Here's how the part is built. I have some questions about the finished solid (model axes, mm). A direction names the side the tool comes from. Give positions to 0.01 mm unless a question says otherwise; leave off trailing zeros. Loops run counter-clockwise (first coordinate to the right, second up) from the corner with the lowest first, then second, coordinate; pieces in that order, holes last. Notation, with made-up numbers: (-36, 61) - (-18, 61) arc R23 cw to (-18, 82) - close; hole circle Ø8 at (9, 32). An arc over 180 degrees is marked (long way). Return JSON: item names as keys, results as strings. Group by question number.
(1) On a 3-axis mill with a long thin cutter (end or side, diameter ignored), from which of +Z, -Z, +X, -X, +Y, -Y can I reach the whole of each face in a straight line? I mean faces 5 (the flat face through (-68, 2.736, 9)), 6 (the flat face through (-75, 20, -5.5)), 7 (the flat face through (-70, 21, 15)), 8 (the flat face through (-70, 14.113, 23)), 9 (the flat face through (-72, 15, 18)). Say none if no direction works.
(2) If we section it at C-C (x = -83): Please give me the cut outline in (y, z).
(3) If we section it at A-A (z = 22): Please give me the cut outline in (x, y), then the cut area to 3 significant figures.
(4) If we section it at B-B (z = 16): Please give me the cut outline in (x, y), then the cut area to 3 significant figures.
(5) If we mould it in two halves opening along X, with no side actions, what happens to faces 1 (the flat face through (-65, 20, -5.5)), 2 (the flat face through (-72.3, 12.5, -1.5)), 3 (the flat face through (-73.543, 18, 23)), 4 (the cylindrical face through (-70.06, 12.62, 25.28))? For each: released by +X, released by -X, zero draft, split by the parting line, or undercut.
(6) I need wall thicknesses on probe 1 along Z at (x, y) = (-58.5, 15); probe 2 along Z at (x, y) = (-70.5, 17); probe 3 along X at (y, z) = (16, 22.5). Which ranges of each line are inside material? Lowest first, please. Write a range as [from, to].
(7) For P1, Ø6, axis at y = 15.5, z = -1.5, coming from the +X side; P2, Ø2, axis at x = -67, y = 18.5, coming from the -Z side; P3, Ø1.8, axis at y = 4.5, z = 7, coming from the +X side, each with a flat end and sliding along its axis, tell me the tip position at first contact or that it passes through.
(8) If we section it at D-D (x = -65): State how many separate pieces and enclosed holes the cut face has, then the cut area to 3 significant figures.
```python
from build123d import *

# Parameters (mm, degrees)
SALIENTE_EXTRUIR1_DEPTH = 18
SALIENTE_EXTRUIR2_START = 1.5
CROQUIS2_R              = 2.7
SALIENTE_EXTRUIR2_DEPTH = 1.5
SALIENTE_EXTRUIR3_DEPTH = 1.5
CROQUIS6_W              = 5.4
CROQUIS6_H              = 1.803822617
SALIENTE_EXTRUIR7_DEPTH = 10
CROQUIS10_W             = 5.4
CROQUIS10_H             = 10
CORTAR_EXTRUIR3_DEPTH   = 10
CROQUIS12_W             = 50.345864286
CROQUIS12_H             = 43.398115734
CORTAR_EXTRUIR4_DEPTH   = 30
CROQUIS14_W             = 2
CROQUIS14_H             = 3
CORTAR_EXTRUIR5_DEPTH   = 30
CORTAR_EXTRUIR7_START   = -7.4
CROQUIS16_W             = 3
CROQUIS16_H             = 7.002646448
CROQUIS16_H_2           = 3.270183245
CORTAR_EXTRUIR7_DEPTH   = 7.4
CROQUIS17_W             = 3.7
CROQUIS17_H             = 3
REVOLUCI_N2_ANGLE       = 180
CROQUIS19_W             = 0.5
CROQUIS19_H             = 9
REVOLUCI_N3_ANGLE       = 180


with BuildPart() as part:
    # Croquis1 → Saliente-Extruir1 (new body)
    with BuildSketch(Plane.XY):
        with BuildLine():
            Line((-53.667784589, 33.4650382), (-54.417784589, 34.764076306))
            Line((-54.417784589, 34.764076306), (-59.613937012, 31.764076306))
            ThreePointArc((-59.613937012, 31.764076306), (-73.945502317, 40.827707086), (-87.584573208, 30.752047693))
            Line((-87.584573208, 30.752047693), (-88.334573208, 29.453009587))
            Line((-88.334573208, 29.453009587), (-83.138420786, 26.453009587))
            ThreePointArc((-83.138420786, 26.453009587), (-83.82197264, 9.509694567), (-68.276660199, 2.735742387))
            Line((-68.276660199, 2.735742387), (-66.776660199, 2.735742387))
            Line((-66.776660199, 2.735742387), (-66.776660199, 8.735742387))
            ThreePointArc((-66.776660199, 8.735742387), (-51.761543041, 16.615426627), (-53.667784589, 33.4650382))
        make_face()
        with BuildLine():
            Line((-54.507549641, 31.745180452), (-55.016343575, 32.626437397))
            Line((-55.016343575, 32.626437397), (-60.212495998, 29.626437397))
            ThreePointArc((-60.212495998, 29.626437397), (-72.508207296, 39.071771198), (-85.675250182, 30.884718699))
            Line((-85.675250182, 30.884718699), (-86.184044116, 30.003461754))
            Line((-86.184044116, 30.003461754), (-80.987891693, 27.003461754))
            ThreePointArc((-80.987891693, 27.003461754), (-83.019935064, 11.632396511), (-69.346218174, 4.322929129))
            Line((-69.346218174, 4.322929129), (-68.328630306, 4.322929129))
            Line((-68.328630306, 4.322929129), (-68.328630306, 10.322929129))
            ThreePointArc((-68.328630306, 10.322929129), (-54.000875637, 16.248660571), (-54.507549641, 31.745180452))
        make_face(mode=Mode.SUBTRACT)
    extrude(amount=SALIENTE_EXTRUIR1_DEPTH)

    # Croquis2 → Saliente-Extruir2 (add)
    with BuildSketch(Plane(origin=(0, 0, 0), x_dir=(-1, 0, 0), z_dir=(0, 0, -1)).offset(SALIENTE_EXTRUIR2_START)):
        with BuildLine():
            Line((87.584573208, 30.752047693), (88.334573208, 29.453009587))
            Line((88.334573208, 29.453009587), (83.138420786, 26.453009587))
            ThreePointArc((83.138420786, 26.453009587), (83.82197264, 9.509694567), (68.276660199, 2.735742387))
            Line((68.276660199, 2.735742387), (66.776660199, 2.735742387))
            Line((66.776660199, 2.735742387), (66.776660199, 8.735742387))
            ThreePointArc((66.776660199, 8.735742387), (51.761543041, 16.615426627), (53.667784589, 33.4650382))
            Line((53.667784589, 33.4650382), (54.417784589, 34.764076306))
            Line((54.417784589, 34.764076306), (59.613937012, 31.764076306))
            ThreePointArc((59.613937012, 31.764076306), (73.945502317, 40.827707086), (87.584573208, 30.752047693))
        make_face()
        with Locations((69.843005999, 22.317609427)):
            Circle(CROQUIS2_R, mode=Mode.SUBTRACT)
    extrude(amount=-SALIENTE_EXTRUIR2_DEPTH)

    # Croquis3 → Saliente-Extruir3 (add)
    with BuildSketch(Plane.XY.offset(18)):
        with BuildLine():
            Line((-66.776660199, 8.735742387), (-66.776660199, 2.735742387))
            Line((-66.776660199, 2.735742387), (-68.276660199, 2.735742387))
            ThreePointArc((-68.276660199, 2.735742387), (-83.82197264, 9.509694567), (-83.138420786, 26.453009587))
            Line((-83.138420786, 26.453009587), (-88.334573208, 29.453009587))
            Line((-88.334573208, 29.453009587), (-87.584573208, 30.752047693))
            ThreePointArc((-87.584573208, 30.752047693), (-73.945502317, 40.827707086), (-59.613937012, 31.764076306))
            Line((-59.613937012, 31.764076306), (-54.417784589, 34.764076306))
            Line((-54.417784589, 34.764076306), (-53.667784589, 33.4650382))
            ThreePointArc((-53.667784589, 33.4650382), (-51.761543041, 16.615426627), (-66.776660199, 8.735742387))
        make_face()
    extrude(amount=SALIENTE_EXTRUIR3_DEPTH)

    # Croquis6 → Saliente-Extruir7 (add)
    with BuildSketch(Plane(origin=(0, 0, -1.5), x_dir=(-1, 0, 0), z_dir=(0, 0, -1))):
        with Locations((69.843005999, 21.415698119)):
            Rectangle(CROQUIS6_W, CROQUIS6_H)
    extrude(amount=SALIENTE_EXTRUIR7_DEPTH)

    # Croquis10 → Cortar-Extruir3 (cut)
    with BuildSketch(Plane(origin=(0, 22.317609427, 0), x_dir=(1, 0, 0), z_dir=(0, 1, 0))):
        with Locations((-69.843005999, 6.5)):
            Rectangle(CROQUIS10_W, CROQUIS10_H)
    extrude(amount=-CORTAR_EXTRUIR3_DEPTH, mode=Mode.SUBTRACT)

    # Croquis11 → Revolución1 (revolve)
    with BuildSketch(Plane(origin=(0, 22.317609427, 0), x_dir=(1, 0, 0), z_dir=(0, 1, 0)), mode=Mode.PRIVATE) as revoluci_n1_sk:
        Polygon((-72.543005999, 1.5), (-79.543005999, 1.5), (-72.543005999, 11.5), align=None)
        Polygon((-71.193005999, -19.5), (-69.843005999, -19.5), (-69.843005999, -26.5), (-71.193005999, -26.5), (-79.543005999, -26.5), (-79.543005999, -19.5), align=None)
    revolve(revoluci_n1_sk.sketch.rotate(Axis((-69.843005999, 22.317609427, 19.5), (0, 0, 1)), 180), axis=Axis((-69.843005999, 22.317609427, 19.5), (0, 0, 1)))

    # Croquis12 → Cortar-Extruir4 (cut)
    with BuildSketch(Plane(origin=(0, 22.317609427, 0), x_dir=(1, 0, 0), z_dir=(0, 1, 0))):
        with Locations((-66.462924906, -7.850212976)):
            Rectangle(CROQUIS12_W, CROQUIS12_H)
    extrude(amount=CORTAR_EXTRUIR4_DEPTH, mode=Mode.SUBTRACT)

    # Croquis14 → Cortar-Extruir5 (cut)
    with BuildSketch(Plane(origin=(0, 22.317609427, 0), x_dir=(-1, 0, 0), z_dir=(0, 1, 0))):
        with Locations((65.143005999, -4)):
            Rectangle(CROQUIS14_W, CROQUIS14_H)
        with Locations((74.543005999, -4)):
            Rectangle(CROQUIS14_W, CROQUIS14_H)
        with Locations((74.543005999, 23)):
            Rectangle(CROQUIS14_W, CROQUIS14_H)
        with Locations((65.143005999, 23)):
            Rectangle(CROQUIS14_W, CROQUIS14_H)
    extrude(amount=-CORTAR_EXTRUIR5_DEPTH, mode=Mode.SUBTRACT)

    # Croquis16 → Cortar-Extruir7 (cut)
    with BuildSketch(Plane.ZY.offset(73.543005999).offset(CORTAR_EXTRUIR7_START)):
        with Locations((-4, 12.992198291)):
            Rectangle(CROQUIS16_W, CROQUIS16_H)
        with Locations((23, 12.478250621)):
            Rectangle(CROQUIS16_W, CROQUIS16_H_2)
    extrude(amount=CORTAR_EXTRUIR7_DEPTH, mode=Mode.SUBTRACT)

    # Croquis17 → Revolución2 (revolve)
    with BuildSketch(Plane(origin=(0, 22.317609427, 0), x_dir=(1, 0, 0), z_dir=(0, 1, 0))):
        with Locations((-67.993005999, -16.5)):
            Rectangle(CROQUIS17_W, CROQUIS17_H)
    revolve(axis=Axis((-69.843005999, 22.317609427, 15), (0, 0, -1)), revolution_arc=REVOLUCI_N2_ANGLE)

    # Croquis19 → Revolución3 (revolve)
    with BuildSketch(Plane(origin=(0, 22.317609427, 0), x_dir=(1, 0, 0), z_dir=(0, 1, 0))):
        with Locations((-67.393005999, 7)):
            Rectangle(CROQUIS19_W, CROQUIS19_H)
    revolve(axis=Axis((-69.843005999, 22.317609427, 0), (0, 0, -1)), revolution_arc=REVOLUCI_N3_ANGLE)


solid = part.part
```
Values:
{
 "1": {"face 5": "+Z, -Z, +X, -Y", "face 6": "+Y, -Y", "face 7": "+Y", "face 8": "+X, -X, -Y", "face 9": "none"},
 "2": {"outline": "(8.33, -1.5) - (22.32, -1.5) - (22.32, 0) - (11.59, 0) - (11.59, 18) - (22.32, 18) - (22.32, 19.5) - (8.33, 19.5) - close"},
 "3": {"outline": "(-79.54, 22.32) arc R9.7 ccw to (-75.54, 14.47) - (-75.54, 22.32) - close; (-73.54, 14.11) - (-66.14, 14.11) - (-66.14, 22.32) - (-73.54, 22.32) - close; (-64.14, 14.47) arc R9.7 ccw to (-60.14, 22.32) - (-64.14, 22.32) - close", "area": "105 mm2"},
 "4": {"outline": "(-85.31, 22.32) arc R15.01 ccw to (-68.28, 2.74) - (-66.78, 2.74) - (-66.78, 8.74) arc R15.01 ccw to (-50.07, 22.32) - (-51.89, 22.32) arc R13.62 cw to (-68.33, 10.32) - (-68.33, 4.32) - (-69.35, 4.32) arc R13.62 cw to (-83.77, 22.32) - close; (-73.54, 22.32) arc R3.7 ccw to (-66.14, 22.32) - close", "area": "121 mm2"},
 "5": {"face 1": "undercut", "face 2": "zero draft", "face 3": "undercut", "face 4": "split by the parting line"},
 "6": {"probe 1": "[-1.5, 0], [18, 19.5]", "probe 2": "[-7.7, 0], [18, 26.5]", "probe 3": "[-77.2, -75.54], [-73.54, -66.14], [-64.14, -62.48]"},
 "7": {"P1": "x = -50.92", "P2": "z = -9.99", "P3": "x = -66.78"},
 "8": {"separate pieces": "3", "enclosed holes": "0", "area": "117 mm2"}
}
